The model under review builds one solid part; all positions refer to its coordinate system, in mm. A direction names the side the tool comes from. Round coordinates to 2 decimals unless told otherwise and drop trailing zeros. Order: outer loops, then holes, each group sorted by start corner. A loop starts at its lowest first (then second) coordinate and runs counter-clockwise, first axis right, second up. Notation, with made-up numbers: (46.25, 44) -> (50.25, 44) arc R26 ccw to (50.25, 79) -> close; hole circle Ø5 at (69.25, 33). An arc over 180 degrees is marked (long way). Return JSON: item names as keys, results as strings. Group by question number.
from build123d import *
from OCP.BRepFilletAPI import BRepFilletAPI_MakeChamfer

# Parameters (mm, degrees)
BOSS_EXTRUDE1_DEPTH   = 25.4
SKETCH2_W             = 11.049
SKETCH2_H             = 44.45
BOSS_EXTRUDE2_DEPTH   = 52.324
CHAMFER1_SIZE         = 6.35
F_1_12_TAPPED_HOLE1_D = 23.41626
CHAMFER2_SIZE         = 15.24
CHAMFER2_SIZE2        = 8.798818102
SKETCH5_W             = 31.303655522
SKETCH5_H             = 45.499968027
CUT_EXTRUDE1_DEPTH    = 19.05
BOSS_EXTRUDE3_REACH   = 98.264
SKETCH6_R             = 25.4
BOSS_EXTRUDE4_START   = -50.8
SKETCH6_2_R           = 25.4
BOSS_EXTRUDE4_DEPTH   = 11.049
SKETCH7_R             = 12.954
CUT_EXTRUDE2_DEPTH    = 118.730027504
CHAMFER4_SIZE         = 5.08
CHAMFER4_SIZE2        = 2.932939367


with BuildPart() as part:
    # Sketch1 → Boss-Extrude1 (new body)
    with BuildSketch(Plane(origin=(0, 0, 0), x_dir=(1, 0, 0), z_dir=(0, 1, 0))):
        with BuildLine():
            Line((-25.4, -22.225), (-12.296722124, -22.225))
            ThreePointArc((-12.296722124, -22.225), (0, -25.4), (12.296722124, -22.225))
            Line((12.296722124, -22.225), (25.4, -22.225))
            Line((25.4, -22.225), (25.4, 22.225))
            Line((25.4, 22.225), (12.296722124, 22.225))
            ThreePointArc((12.296722124, 22.225), (0, 25.4), (-12.296722124, 22.225))
            Line((-12.296722124, 22.225), (-25.4, 22.225))
            Line((-25.4, 22.225), (-25.4, -22.225))
        make_face()
    extrude(amount=BOSS_EXTRUDE1_DEPTH)

    # Sketch2 → Boss-Extrude2 (add)
    with BuildSketch(Plane(origin=(0, 25.4, 0), x_dir=(1, 0, 0), z_dir=(0, 1, 0))):
        with Locations((-19.8755, 0)):
            Rectangle(SKETCH2_W, SKETCH2_H)
        with Locations((19.8755, 0)):
            Rectangle(SKETCH2_W, SKETCH2_H)
    extrude(amount=BOSS_EXTRUDE2_DEPTH)

    # Chamfer1
    chamfer1_edges = [part.edges().sort_by_distance(p)[0] for p in [
        (0, 25.4, 25.4),
        (13.323861062, 25.4, 22.225),
        (-13.323861062, 25.4, 22.225),
        (13.323861062, 25.4, -22.225),
        (0, 25.4, -25.4),
        (-13.323861062, 25.4, -22.225),
    ]]
    chamfer(chamfer1_edges, length=CHAMFER1_SIZE)

    # 1-12 Tapped Hole1 (through all)
    with Locations(Plane(origin=(0, 0, 0), x_dir=(-1, 0, 0), z_dir=(0, -1, 0))):
        with Locations((0, 0)):
            Hole(F_1_12_TAPPED_HOLE1_D / 2)

    # Chamfer2: one chamfer whose edges measure the first distance from different faces: ONE call of the kernel's chamfer builder (chamfer() names one face for all edges)
    chamfer2_edges_1 = [part.edges().sort_by_distance(p)[0] for p in [
        (25.4, 38.862, -22.225),
        (25.4, 38.862, 22.225),
    ]]
    chamfer2_side_1 = [part.faces().sort_by_distance(p)[0] for p in [
        (25.4, 38.862, 0),
    ]]
    chamfer2_edges_2 = [part.edges().sort_by_distance(p)[0] for p in [
        (-25.4, 38.862, 22.225),
        (-25.4, 38.862, -22.225),
    ]]
    chamfer2_side_2 = [part.faces().sort_by_distance(p)[0] for p in [
        (-25.4, 38.862, 0),
    ]]
    chamfer2 = BRepFilletAPI_MakeChamfer(part.part.solid().wrapped)
    for e in chamfer2_edges_1:
        chamfer2.Add(CHAMFER2_SIZE, CHAMFER2_SIZE2, e.wrapped, chamfer2_side_1[0].wrapped)  # the first distance lies on this face
    for e in chamfer2_edges_2:
        chamfer2.Add(CHAMFER2_SIZE, CHAMFER2_SIZE2, e.wrapped, chamfer2_side_2[0].wrapped)  # the first distance lies on this face
    add(Compound.cast(chamfer2.Shape()), mode=Mode.REPLACE)

    # Sketch5 → Cut-Extrude1 (cut)
    with BuildSketch(Plane.XZ):
        with Locations((-37.876827761, -1.94234058)):
            Rectangle(SKETCH5_W, SKETCH5_H)
        with Locations((37.876827761, -1.94234058)):
            Rectangle(SKETCH5_W, SKETCH5_H)
    extrude(amount=-CUT_EXTRUDE1_DEPTH, mode=Mode.SUBTRACT)

    # Boss-Extrude3: up to this face of the body (flat: up to its plane)
    boss_extrude3_end = Plane(part.part.faces().sort_by_distance((14.351, 51.080086798, 0))[0])
    # Sketch6 → Boss-Extrude3 (add, up to the picked face)
    with BuildSketch(Plane(origin=(25.4, 0, 0), x_dir=(0, 0, -1), z_dir=(1, 0, 0)), mode=Mode.PRIVATE) as boss_extrude3_sk1:
        with Locations((0, 77.724)):
            Circle(SKETCH6_R)
    boss_extrude3_tool1 = split(extrude(boss_extrude3_sk1.sketch, amount=-BOSS_EXTRUDE3_REACH, mode=Mode.PRIVATE), bisect_by=boss_extrude3_end, keep=Keep.BOTH, mode=Mode.PRIVATE)
    add(boss_extrude3_tool1.solids().sort_by(Axis((25.4, 77.724, 0), (-1, 0, 0)))[0])

    # Sketch6<2> → Boss-Extrude4 (add)
    with BuildSketch(Plane(origin=(25.4, 0, 0), x_dir=(0, 0, -1), z_dir=(1, 0, 0)).offset(BOSS_EXTRUDE4_START)):
        with Locations((0, 77.724)):
            Circle(SKETCH6_2_R)
    extrude(amount=BOSS_EXTRUDE4_DEPTH)

    # Sketch7 → Cut-Extrude2 (cut, through all)
    with BuildSketch(Plane(origin=(25.4, 0, 0), x_dir=(0, 0, -1), z_dir=(1, 0, 0))):
        with Locations((0, 77.724)):
            Circle(SKETCH7_R)
    extrude(amount=-CUT_EXTRUDE2_DEPTH, mode=Mode.SUBTRACT)

    # Chamfer4: one chamfer whose edges measure the first distance from different faces: ONE call of the kernel's chamfer builder (chamfer() names one face for all edges)
    chamfer4_edges_1 = [part.edges().sort_by_distance(p)[0] for p in [
        (-25.4, 19.05, 0),
    ]]
    chamfer4_side_1 = [part.faces().sort_by_distance(p)[0] for p in [
        (-25.4, 36.176658328, -6.002702821),
    ]]
    chamfer4_edges_2 = [part.edges().sort_by_distance(p)[0] for p in [
        (25.4, 19.05, 0),
    ]]
    chamfer4_side_2 = [part.faces().sort_by_distance(p)[0] for p in [
        (25.4, 102.141702821, 0),
    ]]
    chamfer4 = BRepFilletAPI_MakeChamfer(part.part.solid().wrapped)
    for e in chamfer4_edges_1:
        chamfer4.Add(CHAMFER4_SIZE, CHAMFER4_SIZE2, e.wrapped, chamfer4_side_1[0].wrapped)  # the first distance lies on this face
    for e in chamfer4_edges_2:
        chamfer4.Add(CHAMFER4_SIZE, CHAMFER4_SIZE2, e.wrapped, chamfer4_side_2[0].wrapped)  # the first distance lies on this face
    add(Compound.cast(chamfer4.Shape()), mode=Mode.REPLACE)


solid = part.part
Item 1: Consider section B-B on x = 0. State the section outline as (y, z) points.
Item 2: Consider section D-D on y = 69. State the section outline as (x, z) points, plus the area to 3 significant figures.
Item 3: Insertion check: pin 1 Ø1.5 at (x, y) = (16.5, 41) entering from +Z (3 decimals); pin 2 Ø8 at (x, z) = (17, 10) entering from -Y; pin 3 Ø1.3 at (x, y) = (-13.5, 32) entering from +Z; pin 4 Ø15 at (y, z) = (11, 0) entering from -X (3 decimals). Each pin has a flat end and moves straight along its axis. Give the tip position at first contact, or say it passes through.
Item 4: The part is to be moulded in two halves that separate along X. For faces 5 (the face through (-11.697, 12.878, -0.515)), 6 (the face through (0, 25.4, -13)), 7 (the face through (-25.4, 64, 0)), 8 (the face through (15, 25, 22.225)), say which applies: +X half, -X half, draft (parallel to the pull), parting line (faces both ways), or undercut.
Item 5: For faces 1 (the face through (-12.892, 22.269, 19.006)), 2 (the face through (19.96, 32.26, -16.41)), 3 (the face through (-12.838, 22.181, -19.094)), 4 (the face through (-15, 25, -22.225)), list the 3-axis set-ups (+Z, -Z, +X, -X, +Y, -Y) from which the entire face can be reached by the end or side of a thin tool; tool diameter is ignored.
Item 6: Consider section A-A on y = 30. State the section outline as (x, z) points (3 decimals).
Item 7: Wall thickness on line 1 along Y through (x, z) = (14.5, 0); line 2 along X through (y, z) = (64.5, -16.5); line 3 along X through (y, z) = (55, 22): over which ranges is each line inside the solid? List them lowest first.
Item 8: Consider section C-C on z = 0. State the section outline as (x, y) points (3 decimals), plus the area to 3 significant figures.
Values:
{
 "1": {"outline": "(0, -25.4) -> (19.05, -25.4) -> (25.4, -19.05) -> (25.4, -11.71) -> (0, -11.71) -> close; (0, 11.71) -> (25.4, 11.71) -> (25.4, 19.05) -> (19.05, 25.4) -> (0, 25.4) -> close"},
 "2": {"outline": "(-25.4, -23.85) -> (-14.35, -23.85) -> (-14.35, -9.58) -> (-25.4, -9.58) -> close; (-25.4, 9.58) -> (-14.35, 9.58) -> (-14.35, 23.85) -> (-25.4, 23.85) -> close; (14.35, -23.85) -> (25.4, -23.85) -> (25.4, -9.58) -> (14.35, -9.58) -> close; (14.35, 9.58) -> (25.4, 9.58) -> (25.4, 23.85) -> (14.35, 23.85) -> close", "area": "631 mm^2"},
 "3": {"pin 1": "z = 22.225", "pin 2": "y = 0", "pin 3": "through", "pin 4": "x = -22.225"},
 "4": {"face 5": "undercut", "face 6": "undercut", "face 7": "-X half", "face 8": "draft"},
 "5": {"face 1": "+Z, +Y", "face 2": "-Z, +X, -Y", "face 3": "-Z, +Y", "face 4": "-Z, -X, -Y"},
 "6": {"outline": "(-25.4, -6.985) -> (-16.601, -22.225) -> (-14.351, -22.225) -> (-14.351, 22.225) -> (-16.601, 22.225) -> (-25.4, 6.985) -> close; (14.351, -22.225) -> (16.601, -22.225) -> (25.4, -6.985) -> (25.4, 6.985) -> (16.601, 22.225) -> (14.351, 22.225) -> close"},
 "7": {"line 1": "0 to 64.77, 90.68 to 103.12", "line 2": "-25.4 to -14.35, 14.35 to 25.4", "line 3": "-16.73 to -14.35, 14.35 to 16.73"},
 "8": {"outline": "(-25.4, 24.13) -> (-22.467, 19.05) -> (-22.225, 19.05) -> (-22.225, 0) -> (-11.708, 0) -> (-11.708, 25.4) -> (-14.351, 25.4) -> (-14.351, 64.77) -> (-25.4, 64.77) -> close; (-25.4, 90.678) -> (-14.351, 90.678) -> (-14.351, 103.124) -> (-25.4, 103.124) -> close; (11.708, 0) -> (22.225, 0) -> (22.225, 19.05) -> (22.467, 19.05) -> (25.4, 24.13) -> (25.4, 64.77) -> (14.351, 64.77) -> (14.351, 25.4) -> (11.708, 25.4) -> close; (14.351, 90.678) -> (25.4, 90.678) -> (25.4, 103.124) -> (14.351, 103.124) -> close", "area": "1,700 mm^2"}
}
